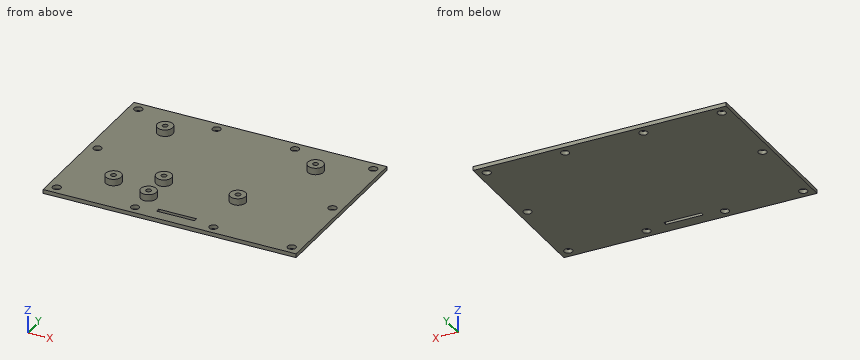
```python
from build123d import *

# Parameters (mm, degrees)
SKETCH1_W           = 195
SKETCH1_H           = 136
SKETCH1_W_2         = 171
SKETCH1_H_2         = 112
SKETCH1_W_3         = 160
SKETCH1_H_3         = 96
BOSS_EXTRUDE1_DEPTH = 1.5
SKETCH1_3_W         = 195
SKETCH1_3_H         = 136
SKETCH1_3_W_2       = 171
SKETCH1_3_H_2       = 112
SKETCH1_3_W_3       = 160
SKETCH1_3_H_3       = 96
BOSS_EXTRUDE2_DEPTH = 1.5
SKETCH2_R           = 3.175
CUT_EXTRUDE1_DEPTH  = 119.908578328
SKETCH3_R           = 6
SKETCH3_R_2         = 2
BOSS_EXTRUDE3_DEPTH = 5.1
SKETCH4_R           = 6
SKETCH4_R_2         = 2
BOSS_EXTRUDE6_DEPTH = 5.1


with BuildPart() as part:
    # Sketch1 → Boss-Extrude1 (new body)
    # profile 1 of 3: a face of its own
    with BuildSketch(Plane.XY):
        Rectangle(SKETCH1_W, SKETCH1_H)
        Polygon((85.5, 56), (85.5, -56), (14.5, -56), (14.5, -59), (-14.5, -59), (-14.5, -56), (-85.5, -56), (-85.5, 56), align=None, mode=Mode.SUBTRACT)
    # profile 2 of 3: a face of its own
    with BuildSketch(Plane.XY):
        Rectangle(SKETCH1_W_2, SKETCH1_H_2)
        with Locations((0, 3)):
            Rectangle(SKETCH1_W_3, SKETCH1_H_3, mode=Mode.SUBTRACT)
    # profile 3 of 3: a face of its own
    with BuildSketch(Plane.XY):
        with Locations((0, 3)):
            Rectangle(SKETCH1_W_3, SKETCH1_H_3)
    extrude(amount=-BOSS_EXTRUDE1_DEPTH)

    # Sketch1_3 → Boss-Extrude2 (add)
    # profile 1 of 3: a face of its own
    with BuildSketch(Plane.XY):
        Rectangle(SKETCH1_3_W, SKETCH1_3_H)
        Polygon((85.5, 56), (85.5, -56), (14.5, -56), (14.5, -59), (-14.5, -59), (-14.5, -56), (-85.5, -56), (-85.5, 56), align=None, mode=Mode.SUBTRACT)
    # profile 2 of 3: a face of its own
    with BuildSketch(Plane.XY):
        Rectangle(SKETCH1_3_W_2, SKETCH1_3_H_2)
        with Locations((0, 3)):
            Rectangle(SKETCH1_3_W_3, SKETCH1_3_H_3, mode=Mode.SUBTRACT)
    # profile 3 of 3: a face of its own
    with BuildSketch(Plane.XY):
        with Locations((0, 3)):
            Rectangle(SKETCH1_3_W_3, SKETCH1_3_H_3)
    extrude(amount=BOSS_EXTRUDE2_DEPTH)

    # Sketch2 → Cut-Extrude1 (cut, through all)
    with BuildSketch(Plane.XY.offset(1.5)):
        with Locations((-90.5, 61)):
            Circle(SKETCH2_R)
        with Locations((90.5, 61)):
            Circle(SKETCH2_R)
        with Locations((90.5, -61)):
            Circle(SKETCH2_R)
        with Locations((-90.5, -61)):
            Circle(SKETCH2_R)
        with Locations((-90.5, 0)):
            Circle(SKETCH2_R)
        with Locations((30.166666667, 61)):
            Circle(SKETCH2_R)
        with Locations((90.5, 0)):
            Circle(SKETCH2_R)
        with Locations((30.166666667, -61)):
            Circle(SKETCH2_R)
        with Locations((-30.166666667, -61)):
            Circle(SKETCH2_R)
        with Locations((-30.166666667, 61)):
            Circle(SKETCH2_R)
    extrude(amount=-CUT_EXTRUDE1_DEPTH, mode=Mode.SUBTRACT)

    # Sketch3 → Boss-Extrude3 (add)
    with BuildSketch(Plane.XY.offset(1.5)):
        with Locations((-28.5, -44)):
            Circle(SKETCH3_R)
        with Locations((-28.5, -44)):
            Circle(SKETCH3_R_2, mode=Mode.SUBTRACT)
    boss_extrude3 = extrude(amount=BOSS_EXTRUDE3_DEPTH)

    # Sketch-Pattern1: Boss-Extrude3 at 2 more places
    with Locations((0, 23, 0), (57, 23, 0)):
        add(boss_extrude3)

    # Sketch4 → Boss-Extrude6 (add)
    with BuildSketch(Plane.XY.offset(1.5)):
        with Locations((-59.585970737, -36.007477459)):
            Circle(SKETCH4_R)
        with Locations((-59.585970737, -36.007477459)):
            Circle(SKETCH4_R_2, mode=Mode.SUBTRACT)
    boss_extrude6 = extrude(amount=BOSS_EXTRUDE6_DEPTH)

    # Sketch-Pattern2: Boss-Extrude6 at 2 more places
    with Locations((0, 77, 0), (116, 77, 0)):
        add(boss_extrude6)


solid = part.part
```
Part model, mm, in its own coordinate system. Coordinates: 2 decimals unless noted, no trailing zeros. Order: outer loops, then holes, each group sorted by start corner. A loop starts at its lowest first (then second) coordinate and runs counter-clockwise, first axis right, second up. Notation, with made-up numbers: (-36.5, -19) -> (9.5, -19) arc R7 cw to (9.5, -7) -> close; hole circle Ø5 at (-17.5, 64). An arc over 180 degrees is marked (long way). Put each result on its own line as item: value. Start each with the question number.
(1) Band-saw the part on D-D (y = -61). Give the cut face in (x, z) (3 decimals).
(2) Probe line 1 along Y through (x, z) = (-90.5, -0.7) (3 decimals); line 2 along Y through (x, z) = (-88, 0.25); line 3 along X through (y, z) = (-56.5, -0.75). List the from-to ranges inside material, lowest first. Write a range as [from, to].
(3) Band-saw the part on C-C (x = 6). Give the cut face in (y, z).
(4) Pin check, flat tips, straight feed: pin 1 Ø3.5 at (x, y) = (-59.59, -36.01) entering from +Z; pin 2 Ø5.5 at (x, y) = (30.17, 61) entering from +Z (3 decimals); pin 3 Ø1 at (y, z) = (-18.5, 3) entering from -X. Stop position of each tip, or through.
(5) Band-saw the part on A-A (x = 90.5). Give the cut face in (y, z) (3 decimals).
(6) Band-saw the part on B-B (y = 0). Give the cut face in (x, z) (3 decimals), then the cut area to 3 significant figures.
Determined:
1. outline: (-97.5, -1.5) -> (-93.675, -1.5) -> (-93.675, 1.5) -> (-97.5, 1.5) -> close; (-87.325, -1.5) -> (-33.342, -1.5) -> (-33.342, 1.5) -> (-87.325, 1.5) -> close; (-26.992, -1.5) -> (26.992, -1.5) -> (26.992, 1.5) -> (-26.992, 1.5) -> close; (33.342, -1.5) -> (87.325, -1.5) -> (87.325, 1.5) -> (33.342, 1.5) -> close; (93.675, -1.5) -> (97.5, -1.5) -> (97.5, 1.5) -> (93.675, 1.5) -> close
2. line 1: y = [-68, -64.175], [-57.825, -3.175], [3.175, 57.825], [64.175, 68]
2. line 2: y = [-68, -62.96], [-59.04, -1.96], [1.96, 59.04], [62.96, 68]
2. line 3: x = [-97.5, -14.5], [14.5, 97.5]
3. outline: (-68, -1.5) -> (-59, -1.5) -> (-59, 1.5) -> (-68, 1.5) -> close; (-56, -1.5) -> (68, -1.5) -> (68, 1.5) -> (-56, 1.5) -> close
4. pin 1: stops at z = 1.5
4. pin 2: passes through
4. pin 3: stops at x = -34.16
5. outline: (-68, -1.5) -> (-64.175, -1.5) -> (-64.175, 1.5) -> (-68, 1.5) -> close; (-57.825, -1.5) -> (-3.175, -1.5) -> (-3.175, 1.5) -> (-57.825, 1.5) -> close; (3.175, -1.5) -> (57.825, -1.5) -> (57.825, 1.5) -> (3.175, 1.5) -> close; (64.175, -1.5) -> (68, -1.5) -> (68, 1.5) -> (64.175, 1.5) -> close
6. outline: (-97.5, -1.5) -> (-93.675, -1.5) -> (-93.675, 1.5) -> (-97.5, 1.5) -> close; (-87.325, -1.5) -> (87.325, -1.5) -> (87.325, 1.5) -> (-87.325, 1.5) -> close; (93.675, -1.5) -> (97.5, -1.5) -> (97.5, 1.5) -> (93.675, 1.5) -> close
6. area: 547 mm²
